Here's how the part is built. I have some questions about the finished solid (model axes, mm). A direction names the side the tool comes from. Coordinates: 2 decimals unless noted, no trailing zeros. Write each loop counter-clockwise with the first axis right and the second up, starting at its lowest first coordinate (ties: lowest second). Pieces come first, ordered by that corner, then holes.
```python
from build123d import *

# Parameters (mm, degrees)
BOSS_EXTRUDE1_DEPTH = 10.922
SKETCH2_W           = 19.05
SKETCH2_H           = 19.05
BOSS_EXTRUDE2_DEPTH = 1.27
SKETCH3_R           = 6.35
CUT_EXTRUDE1_DEPTH  = 6.35
SKETCH4_R           = 1.500000048
CUT_EXTRUDE2_DEPTH  = 1.27
CUT_EXTRUDE3_START  = -1.27
SKETCH5_R           = 1.500000048
CUT_EXTRUDE3_DEPTH  = 1.27


with BuildPart() as part:
    # Sketch1 → Boss-Extrude1 (new body)
    with BuildSketch(Plane.XY):
        with BuildLine():
            Line((2.54, 0), (33.274, 0))
            ThreePointArc((33.274, 0), (35.070051224, 0.743948776), (35.814, 2.54))
            Line((35.814, 2.54), (35.814, 33.274))
            ThreePointArc((35.814, 33.274), (35.070051224, 35.070051224), (33.274, 35.814))
            Line((33.274, 35.814), (2.54, 35.814))
            ThreePointArc((2.54, 35.814), (0.743948776, 35.070051224), (0, 33.274))
            Line((0, 33.274), (0, 2.54))
            ThreePointArc((0, 2.54), (0.743948776, 0.743948776), (2.54, 0))
        make_face()
    extrude(amount=BOSS_EXTRUDE1_DEPTH)

    # Sketch2 → Boss-Extrude2 (add)
    with BuildSketch(Plane.XY.offset(10.922)):
        with Locations((17.990434567, 17.907)):
            Rectangle(SKETCH2_W, SKETCH2_H)
    extrude(amount=BOSS_EXTRUDE2_DEPTH)

    # Sketch3 → Cut-Extrude1 (cut)
    with BuildSketch(Plane.XY.offset(12.192)):
        with Locations((17.990434567, 17.907)):
            Circle(SKETCH3_R)
    extrude(amount=-CUT_EXTRUDE1_DEPTH, mode=Mode.SUBTRACT)

    # Sketch4 → Cut-Extrude2 (cut)
    with BuildSketch(Plane.ZY):
        with Locations((5.461, 17.907)):
            Circle(SKETCH4_R)
    extrude(amount=-CUT_EXTRUDE2_DEPTH, mode=Mode.SUBTRACT)

    # Sketch5 → Cut-Extrude3 (cut)
    with BuildSketch(Plane(origin=(35.814, 0, 0), x_dir=(0, 0, -1), z_dir=(1, 0, 0)).offset(CUT_EXTRUDE3_START)):
        with Locations(Location((-5.461, 17.907, 0), (0, 0, 180))):
            Circle(SKETCH5_R)
    extrude(amount=CUT_EXTRUDE3_DEPTH, mode=Mode.SUBTRACT)


solid = part.part
```
1) We'd pull the mould along Z, two halves only. Please class faces 5 (the face through (0, 18, 3)), 6 (the face through (18, 18, 5.842)), 7 (the face through (34.544, 18, 5)): pulls with the +Z half, pulls with the -Z half, needs draft (parallel to the pull), parting line crosses it, or undercut.
Values follow:
face 5: needs draft
face 6: pulls with the +Z half
face 7: undercut
2) I need wall thicknesses on probe 1 along Z at (x, y) = (5.5, 1); probe 2 along Y at (x, z) = (16.5, 8.75); probe 3 along X at (y, z) = (21.5, 8). Which ranges of each line are inside material? Lowest first, please.
Values follow:
probe 1: z = 0 to 10.92
probe 2: y = 0 to 11.73, 24.08 to 35.81
probe 3: x = 0 to 12.75, 23.23 to 35.81
3) Imagine slicing it at D-D on y = 20. Please give me the cut outline in (x, z).
Values follow:
outline: (0, 0) - (35.81, 0) - (35.81, 10.92) - (27.52, 10.92) - (27.52, 12.19) - (23.99, 12.19) - (23.99, 5.84) - (12, 5.84) - (12, 12.19) - (8.47, 12.19) - (8.47, 10.92) - (0, 10.92) - close
4) On a 3-axis mill with a long thin cutter (end or side, diameter ignored), from which of +Z, -Z, +X, -X, +Y, -Y can I reach the whole of each face in a straight line? I mean faces 1 (the face through (18, 27.432, 12)), 2 (the face through (23.856, 15.475, 9.061)), 3 (the face through (27.515, 18, 12)), 4 (the face through (35.17, 18.482, 6.847)). Say none if no direction works.
Values follow:
face 1: +Z, +X, -X, +Y
face 2: +Z
face 3: +Z, +X, +Y, -Y
face 4: +X
5) Imagine slicing it at A-A on y = 25.5. Please give me the cut outline in (x, z).
Values follow:
outline: (0, 0) - (35.81, 0) - (35.81, 10.92) - (27.52, 10.92) - (27.52, 12.19) - (8.47, 12.19) - (8.47, 10.92) - (0, 10.92) - close
6) Imagine slicing it at C-C on x = 18. Please give me the cut outline in (y, z), then the cut area to 3 significant figures.
Values follow:
outline: (0, 0) - (35.81, 0) - (35.81, 10.92) - (27.43, 10.92) - (27.43, 12.19) - (24.26, 12.19) - (24.26, 5.84) - (11.56, 5.84) - (11.56, 12.19) - (8.38, 12.19) - (8.38, 10.92) - (0, 10.92) - close
area: 335 mm2
7) Will these pins go through, and if not, where does the flat tip stop? pin 1 (10.5 mm diameter, centred on x = 22, y = 22.5, fed in from +Z); pin 2 (0.9 mm diameter, centred on y = 17.5, z = 5.5, fed in from -X); pin 3 (4 mm diameter, centred on x = 19.5, y = 17.5, fed in from +Z); pin 4 (1 mm diameter, centred on y = 17.5, z = 12, fed in from -X).
Values follow:
pin 1: stops at z = 12.19
pin 2: stops at x = 1.27
pin 3: stops at z = 5.84
pin 4: stops at x = 8.47
8) Imagine slicing it at B-B on z = 8. Please give me the cut outline in (x, y).
Values follow:
outline: (0, 2.54) arc R2.54 ccw to (2.54, 0) - (33.27, 0) arc R2.54 ccw to (35.81, 2.54) - (35.81, 33.27) arc R2.54 ccw to (33.27, 35.81) - (2.54, 35.81) arc R2.54 ccw to (0, 33.27) - close; hole circle Ø12.7 at (17.99, 17.91)
